```python
from build123d import *

# Parameters (mm, degrees)
CROQUIS2_R              = 1.75
CROQUIS2_R_2            = 12
SALIENTE_EXTRUIR1_DEPTH = 6.35
REDONDEO1_R             = 3


with BuildPart() as part:
    # Croquis2 → Saliente-Extruir1 (new body)
    with BuildSketch(Plane.XY):
        Polygon((-27.5, -30.5), (97.5, -30.5), (97.5, -14.5), (26.5, -14.5), (26.5, 13.5), (-27.5, 13.5), align=None)
        with Locations((-16, 7)):
            Circle(CROQUIS2_R, mode=Mode.SUBTRACT)
        with Locations((15, 7)):
            Circle(CROQUIS2_R, mode=Mode.SUBTRACT)
        with Locations((15, -24)):
            Circle(CROQUIS2_R, mode=Mode.SUBTRACT)
        with Locations((-16, -24)):
            Circle(CROQUIS2_R, mode=Mode.SUBTRACT)
        with Locations((-0.5, -8.5)):
            Circle(CROQUIS2_R_2, mode=Mode.SUBTRACT)
        with BuildLine():
            Line((71.5, -23.26), (89.5, -23.26))
            ThreePointArc((89.5, -23.26), (92, -25.76), (89.5, -28.26))
            Line((89.5, -28.26), (71.5, -28.26))
            ThreePointArc((71.5, -28.26), (69, -25.76), (71.5, -23.26))
        make_face(mode=Mode.SUBTRACT)
        with BuildLine():
            Line((53.5, -23.26), (35.5, -23.26))
            ThreePointArc((35.5, -23.26), (33, -25.76), (35.5, -28.26))
            Line((35.5, -28.26), (53.5, -28.26))
            ThreePointArc((53.5, -28.26), (56, -25.76), (53.5, -23.26))
        make_face(mode=Mode.SUBTRACT)
    extrude(amount=SALIENTE_EXTRUIR1_DEPTH)

    # Redondeo1
    redondeo1_edges = [part.edges().sort_by_distance(p)[0] for p in [
        (-27.5, 13.5, 3.175),
        (26.5, 13.5, 3.175),
        (26.5, -14.5, 3.175),
        (97.5, -14.5, 3.175),
    ]]
    fillet(redondeo1_edges, radius=REDONDEO1_R)


solid = part.part
```
The listing builds one solid part. Answer for the finished solid, in the listing's coordinates (mm). A direction names the side the tool comes from. Round coordinates to 2 decimals unless told otherwise and drop trailing zeros. Write each loop counter-clockwise with the first axis right and the second up, starting at its lowest first coordinate (ties: lowest second). Pieces come first, ordered by that corner, then holes. Notation, with made-up numbers: (40.5, 6) -> (93.5, 6) arc R21 ccw to (93.5, 43) -> close; hole circle Ø8 at (5.5, 53.25). An arc over 180 degrees is marked (long way). Use CSV: the item, a comma, the result in double quotes. Start each with the question number.
(1) The mould has two halves that part along X. Classify faces 1 (the face through (62, -14.5, 3)), 2 (the face through (97.5, -24, 3)), 3 (the face through (33, -25.7, 3.1)), 4 (the face through (92, -25.7, 3.1)): released by +X, released by -X, zero draft, split by the parting line, or undercut.
(2) Consider L1, parallel to Y at x = 15, z = 3.75; L2, parallel to X at y = -26, z = 5.5; L3, parallel to Y at x = -0.5, z = 3.5. Determine where each line is inside the solid, lowest interval first. Write a range as from..to.
(3) Section D-D on y = -10 is taken. Give the vertices of the cut face in (x, z), then the cut area to 3 significant figures.
(4) Which of the six approach directions +Z, -Z, +X, -X, +Y, -Y give full straight-line access (tool end or side, diameter ignored) to faces 5 (the face through (69, -25.8, 3.1)), 6 (the face through (20, -13, 0)), 7 (the face through (26.5, -1, 3))?
(5) Each of these flat-tipped pins is pushed along its axis until it touches: pin 1 (3 mm diameter, centred on x = 82.5, z = 3.5, fed in from +Y); pin 2 (3 mm diameter, centred on y = -7.5, z = 2.5, fed in from +X). Where does it stop, or does it pass through?
(6) Section A-A on x = -16 is taken. Give the vertices of the cut face in (y, z), then the cut area to 3 significant figures.
(7) Section C-C on x = 38.5 is taken. Give the vertices of the cut face in (y, z), then the cut area to 4 significant figures.
(8) Section B-B on z = 4.75 is taken. Give the vertices of the cut face in (x, y), then the cut area to 3 significant figures.
A:
1,face 1,"zero draft"
1,face 2,"released by +X"
1,face 3,"undercut"
1,face 4,"undercut"
2,L1,"y = -30.5..-25.75, -22.25..5.25, 8.75..13.5"
2,L2,"x = -27.5..33.01, 55.99..69.01, 91.99..97.5"
2,L3,"y = -30.5..-20.5, 3.5..13.5"
3,outline,"(-27.5, 0) -> (-12.41, 0) -> (-12.41, 6.35) -> (-27.5, 6.35) -> close; (11.41, 0) -> (26.5, 0) -> (26.5, 6.35) -> (11.41, 6.35) -> close"
3,area,"192 mm²"
4,face 5,"+Z, -Z"
4,face 6,"-Z, +X, -X, +Y, -Y"
4,face 7,"+Z, -Z, +X, +Y"
5,pin 1,"stops at y = -14.5"
5,pin 2,"stops at x = 26.5"
6,outline,"(-30.5, 0) -> (-25.75, 0) -> (-25.75, 6.35) -> (-30.5, 6.35) -> close; (-22.25, 0) -> (5.25, 0) -> (5.25, 6.35) -> (-22.25, 6.35) -> close; (8.75, 0) -> (13.5, 0) -> (13.5, 6.35) -> (8.75, 6.35) -> close"
6,area,"235 mm²"
7,outline,"(-30.5, 0) -> (-28.26, 0) -> (-28.26, 6.35) -> (-30.5, 6.35) -> close; (-23.26, 0) -> (-14.5, 0) -> (-14.5, 6.35) -> (-23.26, 6.35) -> close"
7,area,"69.85 mm²"
8,outline,"(-27.5, -30.5) -> (97.5, -30.5) -> (97.5, -17.5) arc R3 ccw to (94.5, -14.5) -> (29.5, -14.5) arc R3 cw to (26.5, -11.5) -> (26.5, 10.5) arc R3 ccw to (23.5, 13.5) -> (-24.5, 13.5) arc R3 ccw to (-27.5, 10.5) -> close; hole circle Ø3.5 at (-16, -24); hole circle Ø3.5 at (-16, 7); hole circle Ø24 at (-0.5, -8.5); hole circle Ø3.5 at (15, -24); hole circle Ø3.5 at (15, 7); hole (35.5, -28.26) -> (53.5, -28.26) arc R2.5 ccw to (53.5, -23.26) -> (35.5, -23.26) arc R2.5 ccw to start; hole (71.5, -28.26) -> (89.5, -28.26) arc R2.5 ccw to (89.5, -23.26) -> (71.5, -23.26) arc R2.5 ccw to start"
8,area,"2,800 mm²"
